For this review, use the dimensioned drawing (mm, ordinates from the lowest corner) and the shaded views. Give positions to 0.01 mm unless a question says otherwise; leave off trailing zeros. Loops run counter-clockwise (first coordinate to the right, second up) from the corner with the lowest first, then second, coordinate; pieces in that order, holes last. Notation, with made-up numbers: (79.25, 29.5) - (113.25, 29.5) arc R28 ccw to (113.25, 63.5) - close; hole circle Ø2 at (84, 61). An arc over 180 degrees is marked (long way). Write each question's results on one line, items separated by ' | '.
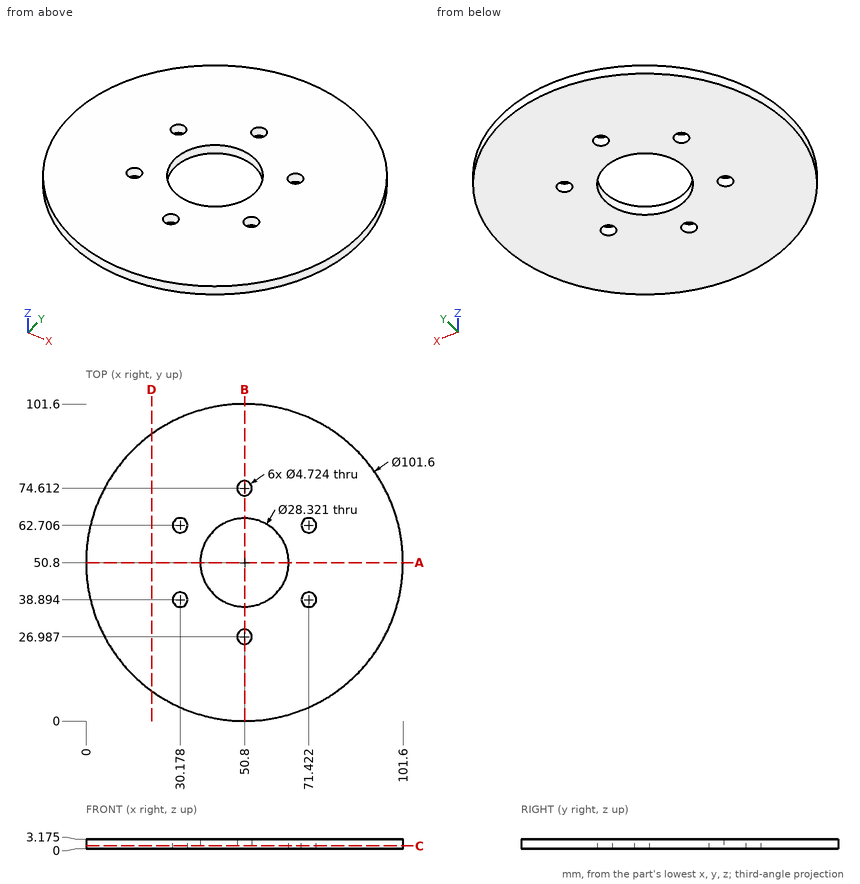
Item 1: We need section A-A on y = 50.8. Give the boundary of the cut face in (x, z) (1 decimal).
Output values:
outline: (0, 0) - (36.6, 0) - (36.6, 3.2) - (0, 3.2) - close; (65, 0) - (101.6, 0) - (101.6, 3.2) - (65, 3.2) - close
Item 2: We need section B-B on x = 50.8. Give the number of separate pieces and of enclosed holes in the cut face, then the cut area to 3 significant figures.
Output values:
separate pieces: 4 | enclosed holes: 0 | area: 203 mm²
Item 3: We need section C-C on z = 0.95. Give the boundary of the cut face in (x, y) (1 decimal), then the cut area to 3 significant figures.
Output values:
outline: circle Ø101.6 at (50.8, 50.8); hole circle Ø4.7 at (30.2, 38.9); hole circle Ø4.7 at (30.2, 62.7); hole circle Ø28.3 at (50.8, 50.8); hole circle Ø4.7 at (50.8, 27); hole circle Ø4.7 at (50.8, 74.6); hole circle Ø4.7 at (71.4, 38.9); hole circle Ø4.7 at (71.4, 62.7) | area: 7,370 mm²
Item 4: We need section D-D on x = 21. Give the boundary of the cut face in (y, z) (1 decimal).
Output values:
outline: (9.7, 0) - (91.9, 0) - (91.9, 3.2) - (9.7, 3.2) - close
Item 5: Wall thickness on probe 1 along X at (y, z) = (50.5, 1.4); probe 2 along Y at (x, z) = (28, 2.55) (1 decimal); probe 3 along Y at (x, z) = (61, 2) (1 decimal): over which ranges is each line inside the solid? List them lowest first.
Output values:
probe 1: x = 0 to 36.64, 64.96 to 101.6 | probe 2: y = 5.4 to 38, 39.8 to 61.8, 63.6 to 96.2 | probe 3: y = 1 to 41, 60.6 to 100.6
